```python
from build123d import *

# Parameters (mm, degrees)
CROQUIS1_W              = 84
CROQUIS1_H              = 150
CROQUIS1_R              = 1.5
CROQUIS1_R_2            = 1.75
SALIENTE_EXTRUIR1_DEPTH = 5


with BuildPart() as part:
    # Croquis1 → Saliente-Extruir1 (new body)
    with BuildSketch(Plane.XY):
        with Locations((42, 75)):
            Rectangle(CROQUIS1_W, CROQUIS1_H)
        with Locations((27, 108)):
            Circle(CROQUIS1_R, mode=Mode.SUBTRACT)
        with Locations((57, 108)):
            Circle(CROQUIS1_R, mode=Mode.SUBTRACT)
        with Locations((16, 139.5)):
            Circle(CROQUIS1_R, mode=Mode.SUBTRACT)
        with Locations((16, 105.5)):
            Circle(CROQUIS1_R, mode=Mode.SUBTRACT)
        with Locations((68, 105.5)):
            Circle(CROQUIS1_R, mode=Mode.SUBTRACT)
        with Locations((68, 139.5)):
            Circle(CROQUIS1_R, mode=Mode.SUBTRACT)
        with Locations((68, 44.5)):
            Circle(CROQUIS1_R, mode=Mode.SUBTRACT)
        with Locations((68, 10.5)):
            Circle(CROQUIS1_R, mode=Mode.SUBTRACT)
        with Locations((16, 10.5)):
            Circle(CROQUIS1_R, mode=Mode.SUBTRACT)
        with Locations((16, 44.5)):
            Circle(CROQUIS1_R, mode=Mode.SUBTRACT)
        with Locations((7, 87)):
            Circle(CROQUIS1_R_2, mode=Mode.SUBTRACT)
        with Locations((24, 87)):
            Circle(CROQUIS1_R_2, mode=Mode.SUBTRACT)
        with Locations((24, 63)):
            Circle(CROQUIS1_R_2, mode=Mode.SUBTRACT)
        with Locations((7, 63)):
            Circle(CROQUIS1_R_2, mode=Mode.SUBTRACT)
        with Locations((60, 63)):
            Circle(CROQUIS1_R_2, mode=Mode.SUBTRACT)
        with Locations((60, 87)):
            Circle(CROQUIS1_R_2, mode=Mode.SUBTRACT)
        with Locations((77, 63)):
            Circle(CROQUIS1_R_2, mode=Mode.SUBTRACT)
        with Locations((77, 87)):
            Circle(CROQUIS1_R_2, mode=Mode.SUBTRACT)
        with Locations((27, 140)):
            Circle(CROQUIS1_R, mode=Mode.SUBTRACT)
        with Locations((57, 140)):
            Circle(CROQUIS1_R, mode=Mode.SUBTRACT)
        with Locations((57, 42)):
            Circle(CROQUIS1_R, mode=Mode.SUBTRACT)
        with Locations((27, 42)):
            Circle(CROQUIS1_R, mode=Mode.SUBTRACT)
        with Locations((57, 10)):
            Circle(CROQUIS1_R, mode=Mode.SUBTRACT)
        with Locations((27, 10)):
            Circle(CROQUIS1_R, mode=Mode.SUBTRACT)
        with BuildLine():
            Line((34.323343601, 80.561599107), (35.636741331, 81.897273116))
            Line((35.636741331, 81.897273116), (37.36006695, 80.894327587))
            ThreePointArc((37.36006695, 80.894327587), (37.710271658, 80.796713171), (38.063524454, 80.882645547))
            ThreePointArc((38.063524454, 80.882645547), (38.605161451, 81.142605955), (39.168546725, 81.351285335))
            ThreePointArc((39.168546725, 81.351285335), (39.475874806, 81.545505215), (39.649132657, 81.865120028))
            Line((39.649132657, 81.865120028), (40.126027071, 83.80117856))
            Line((40.126027071, 83.80117856), (41.999203662, 83.816930268))
            Line((41.999203662, 83.816930268), (42.508589309, 81.889165452))
            ThreePointArc((42.508589309, 81.889165452), (42.687197617, 81.572509513), (42.99774843, 81.38348543))
            ThreePointArc((42.99774843, 81.38348543), (43.564563391, 81.184310005), (44.110495542, 80.933495061))
            ThreePointArc((44.110495542, 80.933495061), (44.465143507, 80.853515486), (44.81365711, 80.957005486))
            Line((44.81365711, 80.957005486), (46.519872501, 81.988790329))
            Line((46.519872501, 81.988790329), (47.85554651, 80.675392598))
            Line((47.85554651, 80.675392598), (46.852600981, 78.952066979))
            ThreePointArc((46.852600981, 78.952066979), (46.754986565, 78.601862272), (46.840918941, 78.248609475))
            ThreePointArc((46.840918941, 78.248609475), (47.10087935, 77.706972479), (47.309558729, 77.143587205))
            ThreePointArc((47.309558729, 77.143587205), (47.503778609, 76.836259124), (47.823393422, 76.663001273))
            Line((47.823393422, 76.663001273), (49.759451954, 76.186106858))
            Line((49.759451954, 76.186106858), (49.775203662, 74.312930268))
            Line((49.775203662, 74.312930268), (47.847438846, 73.803544621))
            ThreePointArc((47.847438846, 73.803544621), (47.530782907, 73.624936313), (47.341758824, 73.3143855))
            ThreePointArc((47.341758824, 73.3143855), (47.142583399, 72.747570539), (46.891768456, 72.201638387))
            ThreePointArc((46.891768456, 72.201638387), (46.81178888, 71.846990422), (46.91527888, 71.49847682))
            Line((46.91527888, 71.49847682), (47.947063723, 69.792261428))
            Line((47.947063723, 69.792261428), (46.633665992, 68.456587419))
            Line((46.633665992, 68.456587419), (44.910340373, 69.459532948))
            ThreePointArc((44.910340373, 69.459532948), (44.560135666, 69.557147364), (44.206882869, 69.471214989))
            ThreePointArc((44.206882869, 69.471214989), (43.665245873, 69.21125458), (43.101860599, 69.002575201))
            ThreePointArc((43.101860599, 69.002575201), (42.794532518, 68.80835532), (42.621274667, 68.488740508))
            Line((42.621274667, 68.488740508), (42.144380253, 66.552681975))
            Line((42.144380253, 66.552681975), (40.271203662, 66.536930268))
            Line((40.271203662, 66.536930268), (39.761818015, 68.464695084))
            ThreePointArc((39.761818015, 68.464695084), (39.583209707, 68.781351023), (39.272658894, 68.970375105))
            ThreePointArc((39.272658894, 68.970375105), (38.705843933, 69.169550531), (38.159911781, 69.420365474))
            ThreePointArc((38.159911781, 69.420365474), (37.805263816, 69.500345049), (37.456750214, 69.396855049))
            Line((37.456750214, 69.396855049), (35.750534822, 68.365070207))
            Line((35.750534822, 68.365070207), (34.414860813, 69.678467937))
            Line((34.414860813, 69.678467937), (35.417806342, 71.401793556))
            ThreePointArc((35.417806342, 71.401793556), (35.515420758, 71.751998264), (35.429488383, 72.10525106))
            ThreePointArc((35.429488383, 72.10525106), (35.343451134, 72.270729543), (35.262211867, 72.438615571))
            ThreePointArc((35.262211867, 72.438615571), (35.261157414, 72.550478141), (35.344779164, 72.624786614))
            Line((35.344779164, 72.624786614), (38.519245985, 73.605484883))
            ThreePointArc((38.519245985, 73.605484883), (44.186794242, 75.155248619), (38.541839298, 76.785388052))
            Line((38.541839298, 76.785388052), (35.305805909, 77.629256147))
            ThreePointArc((35.305805909, 77.629256147), (35.21814086, 77.701438299), (35.216498552, 77.814984441))
            ThreePointArc((35.216498552, 77.814984441), (35.295133958, 77.984773898), (35.378638868, 78.152222148))
            ThreePointArc((35.378638868, 78.152222148), (35.458618444, 78.506870113), (35.355128443, 78.855383716))
            Line((35.355128443, 78.855383716), (34.323343601, 80.561599107))
        make_face(mode=Mode.SUBTRACT)
    extrude(amount=SALIENTE_EXTRUIR1_DEPTH)


solid = part.part
```
Source: CAD feature listing. Evaluate the final solid. Frame: model axes, mm. A direction names the side the tool comes from. Give positions to 0.01 mm unless a question says otherwise; leave off trailing zeros. Order: outer loops, then holes, each group sorted by start corner. A loop starts at its lowest first (then second) coordinate and runs counter-clockwise, first axis right, second up.
(1) Contact query for a flat-ended pin moving along its axis: P1, Ø2, axis at x = 77, y = 63, coming from the +Z side. Output: stop coordinate, or through.
(2) Section query C-C (z = 3.1). State how many separate pieces and enclosed holes the cut face has, plus the area to 3 significant figures.
(3) Section query B-B (y = 87). Return the cut outline in (x, z).
(4) Section query A-A (x = 60). Return the cut outline in (y, z), plus the area to 3 significant figures.
(5) Access query for faces 3 (the face through (41, 0, 2)), 4 (the face through (36.91, 73.11, 2.46)). Directions: +Z, -Z, +X, -X, +Y, -Y. A direction counts if a zero-diameter tool reaches every point of the face in a straight line with its end or side. Return the directions, or none.
(6) Pull-direction query (X, two-part tool) for faces 1 (the face through (41, 76, 5)), 2 (the face through (7.9, 88.5, 2.5)); classes: +X half, -X half, draft (parallel to the pull), parting line (faces both ways), or undercut.
(7) Material intervals for line 1 along X through (y, z) = (108, 2); line 2 along Y through (x, z) = (60, 1); line 3 along Y through (x, z) = (27, 3.25), sorted ascending.
Outcome:
1. P1: passes through
2. separate pieces: 1
2. enclosed holes: 25
2. area: 12,300 mm2
3. outline: (0, 0) - (5.25, 0) - (5.25, 5) - (0, 5) - close; (8.75, 0) - (22.25, 0) - (22.25, 5) - (8.75, 5) - close; (25.75, 0) - (58.25, 0) - (58.25, 5) - (25.75, 5) - close; (61.75, 0) - (75.25, 0) - (75.25, 5) - (61.75, 5) - close; (78.75, 0) - (84, 0) - (84, 5) - (78.75, 5) - close
4. outline: (0, 0) - (61.25, 0) - (61.25, 5) - (0, 5) - close; (64.75, 0) - (85.25, 0) - (85.25, 5) - (64.75, 5) - close; (88.75, 0) - (150, 0) - (150, 5) - (88.75, 5) - close
4. area: 715 mm2
5. face 3: +Z, -Z, +X, -X, -Y
5. face 4: +Z, -Z
6. face 1: draft
6. face 2: undercut
7. line 1: x = 0 to 25.5, 28.5 to 55.5, 58.5 to 84
7. line 2: y = 0 to 61.25, 64.75 to 85.25, 88.75 to 150
7. line 3: y = 0 to 8.5, 11.5 to 40.5, 43.5 to 106.5, 109.5 to 138.5, 141.5 to 150
